Geometry: final body of the model. Coordinates: model frame, mm. A direction names the side the tool comes from. Give positions to 0.01 mm unless a question says otherwise; leave off trailing zeros. Order: outer loops, then holes, each group sorted by start corner. A loop starts at its lowest first (then second) coordinate and runs counter-clockwise, first axis right, second up. Notation, with made-up numbers: (13, 50) -> (37, 50) arc R3 cw to (37, 54) -> close; hole circle Ø6 at (50.5, -0.5). An arc over 180 degrees is marked (long way). Write item = value, one per line.
```python
from build123d import *

# Parameters (mm, degrees)
BOSS_EXTRUDE1_DEPTH     = 25.4
BOSS_EXTRUDE1_2_DEPTH   = 25.4
CUT_EXTRUDE1_DEPTH      = 281.867791968
CUT_EXTRUDE1_DEPTH_BACK = 281.867791968
SKETCH2_W               = 46.910236734
SKETCH2_H               = 46.937556504
CUT_EXTRUDE2_DEPTH      = 281.278275978
CUT_EXTRUDE2_DEPTH_BACK = 281.278275978


with BuildPart() as part:
    # Sketch1 → Boss-Extrude1 (new body)
    with BuildSketch(Plane(origin=(0, 0, 0), x_dir=(1, 0, 0), z_dir=(0, 1, 0))):
        with BuildLine():
            Line((0, 80.02759766), (0, 219.067642019))
            Line((0, 219.067642019), (103.040086398, 219.067642019))
            Line((103.040086398, 219.067642019), (103.040086398, 195.999460881))
            Line((103.040086398, 195.999460881), (23.011829096, 195.999460881))
            Line((23.011829096, 195.999460881), (23.011829096, 161.013213822))
            ThreePointArc((23.011829096, 161.013213822), (101.985495584, 126.901824422), (136.744902109, 48.211224327))
            ThreePointArc((136.744902109, 48.211224327), (146.280346481, 62.911008862), (150.026111113, 80.02759766))
            Line((150.026111113, 80.02759766), (150.026111113, 148.011746996))
            Line((150.026111113, 148.011746996), (172.974333949, 148.011746996))
            Line((172.974333949, 148.011746996), (172.974333949, 80.02759766))
            ThreePointArc((172.974333949, 80.02759766), (86.487166974, 0.037389651), (0, 80.02759766))
        make_face()
        with BuildLine():
            Line((23.011829096, 136.058182002), (23.011829096, 80.02759766))
            ThreePointArc((23.011829096, 80.02759766), (54.48283159, 31.69310754), (112.066438029, 28.410547154))
            ThreePointArc((112.066438029, 28.410547154), (90.841729512, 101.512108787), (23.011829096, 136.058182002))
        make_face(mode=Mode.SUBTRACT)
    extrude(amount=BOSS_EXTRUDE1_DEPTH)

    # Sketch3 → Cut-Extrude2 (cut, two sides: drawn at the far end of the back side and taken through both)
    with BuildSketch(Plane(origin=(0, 25.4, 0), x_dir=(1, 0, 0), z_dir=(0, 1, 0)).offset(-CUT_EXTRUDE2_DEPTH_BACK)):
        with BuildLine():
            Line((23.011829096, 161.013213822), (23.011829096, 136.058182002))
            ThreePointArc((23.011829096, 136.058182002), (90.841729512, 101.512108787), (112.066438029, 28.410547154))
            ThreePointArc((112.066438029, 28.410547154), (125.345033885, 37.140114863), (136.744902109, 48.211224327))
            ThreePointArc((136.744902109, 48.211224327), (101.985495584, 126.901824422), (23.011829096, 161.013213822))
        make_face()
    extrude(amount=CUT_EXTRUDE2_DEPTH + CUT_EXTRUDE2_DEPTH_BACK, mode=Mode.SUBTRACT)


with BuildPart() as body_2:
    # Sketch1 → Boss-Extrude1 2 (new body)
    with BuildSketch(Plane(origin=(0, 0, 0), x_dir=(1, 0, 0), z_dir=(0, 1, 0))):
        Polygon((173.927929859, 172.130085515), (150.026111113, 172.130085515), (150.026111113, 195.999460881), (127.017693125, 195.999460881), (127.017693125, 219.067642019), (173.927929859, 219.067642019), align=None)
    extrude(amount=BOSS_EXTRUDE1_2_DEPTH)

    # Sketch2 → Cut-Extrude1 (cut, two sides: drawn at the far end of the back side and taken through both)
    with BuildSketch(Plane(origin=(0, 25.4, 0), x_dir=(1, 0, 0), z_dir=(0, 1, 0)).offset(-CUT_EXTRUDE1_DEPTH_BACK)):
        with Locations((150.472811492, 195.598863767)):
            Rectangle(SKETCH2_W, SKETCH2_H)
    extrude(amount=CUT_EXTRUDE1_DEPTH + CUT_EXTRUDE1_DEPTH_BACK, mode=Mode.SUBTRACT)


solid = part.part
```
1) Section query C-C (x = 88.5). Output: boundary loops of the cut face in (y, z).
Check sheet entries:
outline = (0, -219.07) -> (25.4, -219.07) -> (25.4, -196) -> (0, -196) -> close; (0, -23.11) -> (25.4, -23.11) -> (25.4, -0.06) -> (0, -0.06) -> close
2) Reachability of faces 1 (the face through (64, 13, -195.999)), 2 (the face through (53.76, 12.52, -32.12)), 3 (the face through (125.17, 12.52, -37)) from +Z, -Z, +X, -X, +Y, -Y: full face, straight path, thin tool, end or side. Return the list, or none.
Check sheet entries:
face_1 = +X, +Y, -Y
face_2 = +Y, -Y
face_3 = -Z, +Y, -Y
3) Section query A-A (z = -91.5). Output: boundary loops of the cut face in (x, y).
Check sheet entries:
outline = (0, 0) -> (23.01, 0) -> (23.01, 25.4) -> (0, 25.4) -> close; (150.03, 0) -> (172.97, 0) -> (172.97, 25.4) -> (150.03, 25.4) -> close
4) Line query: line 1 (X direction, y = 11, z = -90); line 2 (Z direction, x = 85.5, y = 6.25); line 3 (Z direction, x = 67, y = 14.5). Output: solid intervals per line, ascending. Write a range as from..to.
Check sheet entries:
line_1 = 0..23.01, 150.03..172.97
line_2 = -219.07..-196, -23.09..-0.04
line_3 = -219.07..-196, -26.13..-2.25
5) Section query B-B (y = 6.75). Output: boundary loops of the cut face in (x, z), plus the area to 3 significant figures.
Check sheet entries:
outline = (0, -219.07) -> (103.04, -219.07) -> (103.04, -196) -> (23.01, -196) -> (23.01, -80.03) arc R63.88 cw to (112.07, -28.41) arc R84.12 cw to (136.74, -48.21) arc R48.93 cw to (150.03, -80.03) -> (150.03, -148.01) -> (172.97, -148.01) -> (172.97, -80.03) arc R86.75 ccw to (0, -80.03) -> close
area = 11,700 mm²
6) First-contact query: P1, Ø7, axis at x = 165.5, y = 8.5, coming from the -Z side; P2, Ø8, axis at x = 57.5, y = 14, coming from the +Z side; P3, Ø3, axis at x = 98, y = 12, coming from the +Z side. Flat tips, straight axial feed; report the tip coordinate or a pass-through.
Check sheet entries:
P1 = -148.01
P2 = -3.71
P3 = -0.62
7) Mould query, pull axis X, two halves, no side actions, for faces 4 (the face through (150.026, 13, -114)), 5 (the face through (88.3, 12.522, -0.056)), 6 (the face through (161, 13, -148.012)). Classes: +X half, -X half, draft (parallel to the pull), parting line (faces both ways), or undercut.
Check sheet entries:
face_4 = undercut
face_5 = parting line
face_6 = draft
8) Section query D-D (z = -162). Output: boundary loops of the cut face in (x, y), plus the area to 4 significant figures.
Check sheet entries:
outline = (0, 0) -> (23.01, 0) -> (23.01, 25.4) -> (0, 25.4) -> close
area = 584.5 mm²
